Verification items for the finished model (mm, model axes). Round coordinates to 2 decimals unless told otherwise and drop trailing zeros. Loops run counter-clockwise (first coordinate to the right, second up) from the corner with the lowest first, then second, coordinate; pieces in that order, holes last. Notation, with made-up numbers: M 57,51 L 94,51 A29 ccw 94,90 Z; hole C 4.5,50.5 d5. An arc over 180 degrees is marked long. One line per item, written item: value.
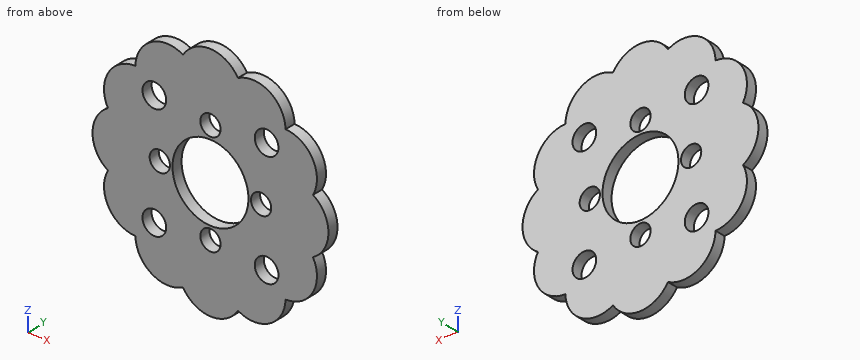
Autodesk Inventor part; units mm, degrees
ref_plane "YZ Plane" through (0, 0, 0) normal (1, 0, 0) x (0, 1, 0)
ref_plane "XZ Plane" through (0, 0, 0) normal (0, 1, 0) x (-1, 0, 0)
ref_plane "XY Plane" through (0, 0, 0) normal (0, 0, 1) x (1, 0, 0)
sketch "Sketch1" plane through (0, 0, 0) normal (0, 1, 0) x (-1, 0, 0)
  circle A0 centre (0, 0) radius 5.625
  circle A1 centre (0, 0) radius 7.5 construction
  circle A2 centre (0, 0) radius 22.225 construction
  circle A3 centre (7.5, 0) radius 1.5
  line L0 (22.225, 0) -> (0, 0) construction
  circle A4 centre (0, 7.5) radius 1.5
  circle A5 centre (-7.5, 0) radius 1.5
  circle A6 centre (0, 0) radius 19.05
  circle A7 centre (0, -7.5) radius 1.5
  point P0 (0, 6)
  point P1 (6, 0)
  point P2 (0, -6)
  point P3 (-6, 0)
  dimension "d1" = 15
  dimension "d2" = 44.45
  dimension "d0" = 11.25
  dimension "d3" = 3
  dimension "d6" = 360
  dimension "d8" = 38.1
extrude "Extrusion1" add sketch "Sketch1" along normal blind 1.5875
sketch "Sketch2" plane through (0, 1.5875, 0) normal (0, 1, 0) x (1, 0, 0)
  circle A0 centre (0, 0) radius 11.75 construction
  line L0 (0, 0) -> (19.05, 0) construction
  circle A1 centre (0, 0) radius 19.05
  line L1 (11.75, 0) -> (0, 0) construction
  line L2 (0, 0) -> (8.3085, -8.3085) construction
  circle A2 centre (8.3085, -8.3085) radius 1.7526
  circle A3 centre (8.3085, 8.3085) radius 1.7526
  circle A4 centre (-8.3085, 8.3085) radius 1.7526
  circle A5 centre (-8.3085, -8.3085) radius 1.7526
  dimension "d11" = 23.5
  dimension "d28" = 45
  dimension "d29" = 3.5052
  dimension "d32" = 360
extrude "Extrusion2" cut sketch "Sketch2" against normal through all contours A2 | A3 | A4 | A5
sketch "Sketch3" plane through (0, 1.5875, 0) normal (0, 1, 0) x (1, 0, 0)
  line L0 (0, 0) -> (12.7, 0) construction
  circle A0 centre (0, 0) radius 12.7 construction
  circle A1 centre (12.7, 0) radius 4.7625
  circle A2 centre (10.9985, 6.35) radius 4.7625
  circle A3 centre (6.35, 10.9985) radius 4.7625
  circle A4 centre (0, 12.7) radius 4.7625
  circle A5 centre (-6.35, 10.9985) radius 4.7625
  circle A6 centre (-10.9985, 6.35) radius 4.7625
  circle A7 centre (-12.7, 0) radius 4.7625
  circle A8 centre (-10.9985, -6.35) radius 4.7625
  circle A9 centre (-6.35, -10.9985) radius 4.7625
  circle A10 centre (0, -12.7) radius 4.7625
  circle A11 centre (6.35, -10.9985) radius 4.7625
  circle A12 centre (10.9985, -6.35) radius 4.7625
  circle A13 centre (0, 0) radius 19.05
  point P0 (11.1112, -11.1112)
  point P1 (4.067, -15.1781)
  point P2 (-4.067, -15.1781)
  point P3 (-11.1112, -11.1112)
  point P4 (-15.1781, -4.067)
  point P5 (-15.1781, 4.067)
  point P6 (-11.1112, 11.1112)
  point P7 (-4.067, 15.1781)
  point P8 (4.067, 15.1781)
  point P9 (11.1112, 11.1112)
  point P10 (15.1781, 4.067)
  point P11 (15.1781, -4.067)
  dimension "d19" = 25.4
  dimension "d20" = 9.525
  dimension "d23" = 360
  dimension "d25" = 38.1
extrude "Extrusion3" cut sketch "Sketch3" against normal blind 25.4
properties part number "Motor Cap" material "Nylon 6/6"
(1) Sectioned sample at D-D on x = 9.5. Enter the section's corners in (y, z), and give its area (3 significant figures).
Completed:
outline: M 0,-14.57 L 1.59,-14.57 L 1.59,-9.59 L 0,-9.59 Z; M 0,-7.02 L 1.59,-7.02 L 1.59,7.02 L 0,7.02 Z; M 0,9.59 L 1.59,9.59 L 1.59,14.57 L 0,14.57 Z
area: 38.1 mm^2
(2) Sectioned sample at A-A on x = 0. Count the separate pieces of the cut face and the enclosed holes in it, and give its area (3 significant figures).
Completed:
separate pieces: 4
enclosed holes: 0
area: 28.1 mm^2
(3) Thickness scan on L1, parallel to Z at x = 0, y = 0.45 (1 decimal); L2, parallel to X at y = 1.4, z = -7; L3, parallel to Z at x = 7.5, y = 1. Record the ranges inside material, lowest first. Write a range as from..to.
Completed:
L1: z = -17.5..-9, -6..-5.6, 5.6..6, 9..17.5
L2: x = -15.72..-9.47, -7.14..-1.41, 1.41..7.14, 9.47..15.72
L3: z = -15.62..-9.86, -6.75..-1.5, 1.5..6.75, 9.86..15.62
